from build123d import *

# Parameters (mm, degrees)
BOSS_EXTRUDE1_DEPTH = 76.2
SKETCH2_R           = 2.9
CUT_EXTRUDE1_DEPTH  = 76.2


with BuildPart() as part:
    # Sketch1 → Boss-Extrude1 (new body)
    with BuildSketch(Plane.XY):
        Polygon((0, 0), (25.4, 0), (25.4, 3.175), (3.175, 3.175), (3.175, 25.4), (0, 25.4), align=None)
    extrude(amount=BOSS_EXTRUDE1_DEPTH)

    # Sketch2 → Cut-Extrude1 (cut)
    with BuildSketch(Plane(origin=(0, 0, 0), x_dir=(1, 0, 0), z_dir=(0, 1, 0))):
        with Locations(Location((14.2875, -25.4, 0), (0, 0, 90))):
            Circle(SKETCH2_R)
        with Locations(Location((14.2875, -50.8, 0), (0, 0, 90))):
            Circle(SKETCH2_R)
    extrude(amount=CUT_EXTRUDE1_DEPTH, mode=Mode.SUBTRACT)


solid = part.part
Here's how the part is built. I have some questions about the finished solid (model axes, mm). A direction names the side the tool comes from. Round coordinates to 2 decimals unless told otherwise and drop trailing zeros. Loops run counter-clockwise (first coordinate to the right, second up) from the corner with the lowest first, then second, coordinate; pieces in that order, holes last.
1. If I drill on line 1 along X through (y, z) = (1.6, 25.4); line 2 along Z through (x, y) = (12.5, 1.75); line 3 along Y through (x, z) = (9.5, 25.5) (3 decimals), over which ranges is the centre line in solid material (lowest first)?
Answer list:
line 1: x = 0 to 11.39, 17.19 to 25.4
line 2: z = 0 to 23.12, 27.68 to 48.52, 53.08 to 76.2
line 3: y = 0 to 3.175
2. If we section it at B-B on x = 15.25: Write out the boundary of the cut face in (y, z) (3 decimals).
Answer list:
outline: (0, 0) - (3.175, 0) - (3.175, 22.664) - (0, 22.664) - close; (0, 28.136) - (3.175, 28.136) - (3.175, 48.064) - (0, 48.064) - close; (0, 53.536) - (3.175, 53.536) - (3.175, 76.2) - (0, 76.2) - close
3. For P1, Ø3, axis at x = 20, z = 59, coming from the +Y side (3 decimals); P2, Ø6.5, axis at y = 15, z = 36.5, coming from the +X side (3 decimals), each with a flat end and sliding along its axis, tell me the tip position at first contact or that it passes through.
Answer list:
P1: stops at y = 3.175
P2: stops at x = 3.175
4. We'd pull the mould along Z, two halves only. Please class faces 1 (the face through (13, 0, 38)), 2 (the face through (15.4, 1.57, 22.72)), 3 (the face through (14.2, 1.6, 53.7)), 4 (the face through (7, 2, 76.2)): +Z half, -Z half, draft (parallel to the pull), parting line (faces both ways), or undercut.
Answer list:
face 1: draft
face 2: undercut
face 3: undercut
face 4: +Z half
5. Which directions (+Z, -Z, +X, -X, +Y, -Y) give clear straight access to the entire face, cutting with the end or side of a thin tool? Please do faces 5 (the face through (0, 13, 38)), 6 (the face through (3.175, 14, 38)).
Answer list:
face 5: +Z, -Z, -X, +Y, -Y
face 6: +Z, -Z, +X, +Y
6. If we section it at A-A on z = 25.4: Write out the boundary of the cut face in (x, y) (1 decimal).
Answer list:
outline: (0, 0) - (11.4, 0) - (11.4, 3.2) - (3.2, 3.2) - (3.2, 25.4) - (0, 25.4) - close; (17.2, 0) - (25.4, 0) - (25.4, 3.2) - (17.2, 3.2) - close
7. If we section it at C-C on y = 13: Write out the boundary of the cut face in (x, z) (3 decimals).
Answer list:
outline: (0, 0) - (3.175, 0) - (3.175, 76.2) - (0, 76.2) - close
